from build123d import *

# Parameters (mm, degrees)
CUT_EXTRUDE1_DEPTH = 0.75
FILLET1_R          = 0.125
WRAP1_START        = -0.125
WRAP1_DEPTH        = 0.125


# Read off the part's stored shape, not the designer's step: Wrap1
with BuildPart() as part:
    # Sketch1 → Revolve1 (revolve)
    with BuildSketch(Plane(origin=(0, 0, 0), x_dir=(0, 0, -1), z_dir=(1, 0, 0)), mode=Mode.PRIVATE) as revolve1_sk:
        with BuildLine():
            Line((0, 1.5), (-1.75, 1.5))
            ThreePointArc((-1.75, 1.5), (-2.334912942, 0.942930354), (-2.75, 0.25))
            Line((-2.75, 0.25), (-2.605662433, 0))
            Line((-2.605662433, 0), (-1.5, 0))
            Line((-1.5, 0), (-1.5, -6))
            Line((-1.5, -6), (0, -6))
            Line((0, -6), (0, 1.5))
        make_face()
    revolve(revolve1_sk.sketch.rotate(Axis((0, -6, 0), (0, 1, 0)), 180), axis=Axis((0, -6, 0), (0, 1, 0)))

    # Sketch2 → Cut-Extrude1 (cut)
    with BuildSketch(Plane(origin=(0, 1.5, 0), x_dir=(1, 0, 0), z_dir=(0, 1, 0))):
        Polygon((0, 1.154700538), (-1, 0.577350269), (-1, -0.577350269), (0, -1.154700538), (1, -0.577350269), (1, 0.577350269), align=None)
    extrude(amount=-CUT_EXTRUDE1_DEPTH, mode=Mode.SUBTRACT)

    # Fillet1
    fillet1_edges = [part.edges().sort_by_distance(p)[0] for p in [
        (0.5, 1.5, -0.866025404),
        (-0.5, 1.5, -0.866025404),
        (-1, 1.5, 0),
        (-0.5, 1.5, 0.866025404),
        (0.5, 1.5, 0.866025404),
        (1, 1.5, 0),
        (0, 1.5, 1.75),
    ]]
    fillet(fillet1_edges, radius=FILLET1_R)

    # Wrap1 outline → Wrap1 (cut)
    with BuildSketch(Plane(origin=(0, 0.75, 0), x_dir=(1, 0, 0), z_dir=(0, 1, 0)).offset(WRAP1_START)):
        with BuildLine():
            add(Edge.make_bspline(
                [(-0.537455829, 0.145072229), (-0.537366548, 0.15735919), (-0.537194747, 0.181002472), (-0.536236546, 0.215136123), (-0.534510696, 0.246473554), (-0.531857696, 0.275057496), (-0.528751002, 0.300937263), (-0.524861231, 0.324098842), (-0.520025531, 0.344486675), (-0.512963856, 0.367808475), (-0.501673714, 0.39403328), (-0.484042302, 0.422215735), (-0.462961845, 0.447719467), (-0.43819726, 0.469796385), (-0.410438674, 0.48826361), (-0.379753396, 0.501330341), (-0.346770262, 0.509472114), (-0.323962243, 0.510388658), (-0.312295573, 0.510857485)],
                knots=[0, 0, 0, 0, 0.075666503, 0.145601872, 0.210267314, 0.268902852, 0.322354979, 0.370758742, 0.413447068, 0.451298193, 0.520734923, 0.588514213, 0.655379256, 0.723813985, 0.792131248, 0.85973193, 0.928250616, 1, 1, 1, 1], degree=3))
            Line((-0.537455829, 0.145072229), (-0.537455829, -0.527604053))
            Line((-0.537455829, -0.527604053), (-0.460532752, -0.527604053))
            Line((-0.460532752, -0.527604053), (-0.460532752, 0.137460049))
            add(Edge.make_bspline(
                [(-0.447712239, 0.305328639), (-0.448774545, 0.301469619), (-0.451134212, 0.292897693), (-0.453525545, 0.278533298), (-0.455753975, 0.261566558), (-0.457491806, 0.241915402), (-0.458861613, 0.219538201), (-0.459832928, 0.194491685), (-0.460431178, 0.166843342), (-0.460497896, 0.147543183), (-0.460532752, 0.137460049)],
                knots=[0, 0, 0, 0, 0.071102967, 0.157938928, 0.258486703, 0.375288845, 0.508476997, 0.656953648, 0.820779591, 1, 1, 1, 1], degree=3))
            add(Edge.make_bspline(
                [(-0.310292367, 0.421113895), (-0.317674297, 0.420714803), (-0.332400851, 0.419918636), (-0.353965955, 0.413875353), (-0.374511474, 0.403804365), (-0.393760239, 0.390026559), (-0.411220155, 0.372905819), (-0.426330799, 0.352966004), (-0.438683838, 0.330213781), (-0.444651659, 0.313764569), (-0.447712239, 0.305328639)],
                knots=[0, 0, 0, 0, 0.115143072, 0.229704239, 0.346728965, 0.47082069, 0.597615275, 0.727089869, 0.860038825, 1, 1, 1, 1], degree=3))
            add(Edge.make_bspline(
                [(-0.17848147, 0.261057806), (-0.178952566, 0.271974178), (-0.179864172, 0.293098195), (-0.186637459, 0.323530756), (-0.198777604, 0.350930356), (-0.212261145, 0.371485038), (-0.225066026, 0.38586534), (-0.235235588, 0.395399384), (-0.246252738, 0.403200746), (-0.257654824, 0.410013084), (-0.269995595, 0.414921405), (-0.282862679, 0.418632696), (-0.296413152, 0.420560449), (-0.305613195, 0.420927309), (-0.310292367, 0.421113895)],
                knots=[0, 0, 0, 0, 0.141583044, 0.273974039, 0.401600231, 0.528456794, 0.591043942, 0.651122908, 0.708825408, 0.765880537, 0.822988251, 0.880580103, 0.939262648, 1, 1, 1, 1], degree=3))
            add(Edge.make_bspline(
                [(-0.340941406, 0.087780562), (-0.334988303, 0.08792105), (-0.323299062, 0.088196907), (-0.306225523, 0.090764835), (-0.289888322, 0.094368098), (-0.274654087, 0.100137271), (-0.260174408, 0.107124777), (-0.24682212, 0.11601785), (-0.234254323, 0.126336142), (-0.222711003, 0.138095802), (-0.212416341, 0.151054166), (-0.203323514, 0.164708223), (-0.195692258, 0.179095557), (-0.189162431, 0.194099224), (-0.184457799, 0.209936522), (-0.181072867, 0.226359939), (-0.178698712, 0.243427453), (-0.178554801, 0.255106579), (-0.17848147, 0.261057806)],
                knots=[0, 0, 0, 0, 0.067065692, 0.131687113, 0.194317921, 0.255289037, 0.314878218, 0.375218702, 0.435653028, 0.497934511, 0.56059698, 0.621980302, 0.682601877, 0.743985199, 0.806139168, 0.868443394, 0.932963888, 1, 1, 1, 1], degree=3))
            Line((-0.340941406, 0.087780562), (-0.357968649, 0.087780562))
            Line((-0.357968649, 0.087780562), (-0.357968649, -0.014783541))
            add(Edge.make_bspline(
                [(-0.152840444, -0.246153733), (-0.152991921, -0.237935238), (-0.153288163, -0.221862292), (-0.155672785, -0.198335348), (-0.159894598, -0.176034257), (-0.165736265, -0.154867378), (-0.173053307, -0.13483662), (-0.182215246, -0.116043494), (-0.192787882, -0.098300128), (-0.20519576, -0.081953022), (-0.21910276, -0.067000398), (-0.234429011, -0.053697294), (-0.25160782, -0.04265632), (-0.269991613, -0.033131715), (-0.29004854, -0.025867397), (-0.311286964, -0.019869429), (-0.334167811, -0.016416131), (-0.349879854, -0.015338382), (-0.357968649, -0.014783541)],
                knots=[0, 0, 0, 0, 0.070899124, 0.138657723, 0.203740428, 0.266496883, 0.327925022, 0.387445969, 0.44662859, 0.505853257, 0.564143059, 0.622569358, 0.680413321, 0.739931479, 0.800819634, 0.864131594, 0.930052902, 1, 1, 1, 1], degree=3))
            add(Edge.make_bspline(
                [(-0.309891726, -0.450680977), (-0.304334961, -0.450571211), (-0.293413044, -0.450355466), (-0.277514036, -0.447340483), (-0.262286727, -0.442989313), (-0.247781817, -0.436676481), (-0.233907442, -0.428733085), (-0.221051475, -0.418678171), (-0.208664071, -0.407189838), (-0.197187775, -0.393882067), (-0.186871623, -0.37903336), (-0.17755536, -0.363253667), (-0.169907305, -0.346235338), (-0.163848892, -0.328206631), (-0.158625475, -0.30926113), (-0.155449196, -0.289102842), (-0.15305503, -0.26797937), (-0.152912733, -0.253506267), (-0.152840444, -0.246153733)],
                knots=[0, 0, 0, 0, 0.057830355, 0.113666545, 0.168061557, 0.222616608, 0.278122197, 0.334218011, 0.392319921, 0.453992458, 0.516935927, 0.58055674, 0.644719566, 0.710965936, 0.778658745, 0.849251577, 0.923417744, 1, 1, 1, 1], degree=3))
            add(Edge.make_bspline(
                [(-0.409250701, -0.417427771), (-0.40035509, -0.422552084), (-0.383473121, -0.432276934), (-0.357561529, -0.44229785), (-0.333383308, -0.449497533), (-0.317482442, -0.450298576), (-0.309891726, -0.450680977)],
                knots=[0, 0, 0, 0, 0.290177362, 0.550694617, 0.785511707, 1, 1, 1, 1], degree=3))
            Line((-0.409250701, -0.417427771), (-0.409250701, -0.507371682))
            add(Edge.make_bspline(
                [(-0.298273137, -0.540424566), (-0.308861639, -0.540097242), (-0.329301798, -0.539465371), (-0.358664913, -0.532954409), (-0.385682425, -0.522833546), (-0.401463988, -0.512480121), (-0.409250701, -0.507371682)],
                knots=[0, 0, 0, 0, 0.269471748, 0.52019112, 0.763259579, 1, 1, 1, 1], degree=3))
            add(Edge.make_bspline(
                [(-0.075917367, -0.249759502), (-0.076128163, -0.26018073), (-0.076541077, -0.280594276), (-0.079227651, -0.310491914), (-0.084396107, -0.33890103), (-0.091033777, -0.365960134), (-0.09992887, -0.391457717), (-0.110563094, -0.41559927), (-0.123397597, -0.438155636), (-0.137962217, -0.459132621), (-0.153934421, -0.478163377), (-0.171095941, -0.494958486), (-0.189740067, -0.508821331), (-0.209271063, -0.520337979), (-0.2298646, -0.529505832), (-0.251686582, -0.535889962), (-0.274626983, -0.539804561), (-0.290311376, -0.540215808), (-0.298273137, -0.540424566)],
                knots=[0, 0, 0, 0, 0.076485505, 0.149823073, 0.219996399, 0.288217649, 0.354082023, 0.417919027, 0.481558234, 0.544225908, 0.605087621, 0.663657146, 0.720011753, 0.77514507, 0.829777395, 0.884976008, 0.941611157, 1, 1, 1, 1], degree=3))
            add(Edge.make_bspline(
                [(-0.194707432, 0.00885428), (-0.185532098, 0.002246917), (-0.167142487, -0.010995852), (-0.14356067, -0.035865532), (-0.123015599, -0.064046821), (-0.106173919, -0.095826321), (-0.092429948, -0.130510752), (-0.082995533, -0.168026939), (-0.077008082, -0.208034101), (-0.076287996, -0.23558107), (-0.075917367, -0.249759502)],
                knots=[0, 0, 0, 0, 0.114174048, 0.228832702, 0.344903554, 0.466103946, 0.591676048, 0.72144281, 0.856626542, 1, 1, 1, 1], degree=3))
            add(Edge.make_bspline(
                [(-0.273032752, 0.036899152), (-0.264977593, 0.035253476), (-0.249714467, 0.032135208), (-0.228666305, 0.025295577), (-0.210172583, 0.018341569), (-0.199638474, 0.011879289), (-0.194707432, 0.00885428)],
                knots=[0, 0, 0, 0, 0.294434237, 0.557901696, 0.79305271, 1, 1, 1, 1], degree=3))
            add(Edge.make_bspline(
                [(-0.200917367, 0.061939216), (-0.205600715, 0.059219735), (-0.215469689, 0.053489114), (-0.232413767, 0.046806913), (-0.251771921, 0.040993346), (-0.265723651, 0.038306664), (-0.273032752, 0.036899152)],
                knots=[0, 0, 0, 0, 0.211315364, 0.445293882, 0.709397831, 1, 1, 1, 1], degree=3))
            add(Edge.make_bspline(
                [(-0.101558393, 0.265064216), (-0.101829728, 0.254158186), (-0.102360461, 0.23282596), (-0.107582885, 0.201794643), (-0.115635878, 0.172523389), (-0.127393107, 0.145424978), (-0.141807851, 0.120566799), (-0.158666737, 0.09801557), (-0.178511599, 0.078390972), (-0.193428545, 0.067437991), (-0.200917367, 0.061939216)],
                knots=[0, 0, 0, 0, 0.138734507, 0.271365083, 0.399463796, 0.524371928, 0.64626696, 0.764603187, 0.881822663, 1, 1, 1, 1], degree=3))
            add(Edge.make_bspline(
                [(-0.312295573, 0.510857485), (-0.304601721, 0.510709635), (-0.289468193, 0.510418818), (-0.267407867, 0.506806308), (-0.246411552, 0.501505665), (-0.226632783, 0.49383833), (-0.208041676, 0.483900131), (-0.190537128, 0.47184286), (-0.174217748, 0.457507541), (-0.159329374, 0.44106616), (-0.145724285, 0.423136003), (-0.133914037, 0.403846519), (-0.123827558, 0.383480477), (-0.115525112, 0.361982783), (-0.109489008, 0.339238969), (-0.104721569, 0.315513437), (-0.102229905, 0.290624502), (-0.101784813, 0.273682609), (-0.101558393, 0.265064216)],
                knots=[0, 0, 0, 0, 0.063537388, 0.124975739, 0.184284437, 0.242302503, 0.299838056, 0.35817297, 0.417627897, 0.478966986, 0.541230446, 0.60342781, 0.66563497, 0.728883988, 0.793562004, 0.859921094, 0.928741429, 1, 1, 1, 1], degree=3))
        make_face()
        Polygon((0.565629107, -0.527604053), (0.583056992, -0.527604053), (0.583056992, 0.472395947), (0.506133915, 0.472395947), (0.506133915, -0.290224246), (-0.016101662, 0.472395947), (-0.032327624, 0.472395947), (-0.032327624, -0.527604053), (0.044595453, -0.527604053), (0.044595453, 0.233012934), align=None)
        Polygon((0.095877504, 0.741626716), (0.244315004, 0.574960049), (0.318633915, 0.574960049), (0.467672376, 0.741626716), (0.350885517, 0.741626716), (0.280172376, 0.662700434), (0.212664363, 0.741626716), align=None)
    extrude(amount=WRAP1_DEPTH, mode=Mode.SUBTRACT)


solid = part.part
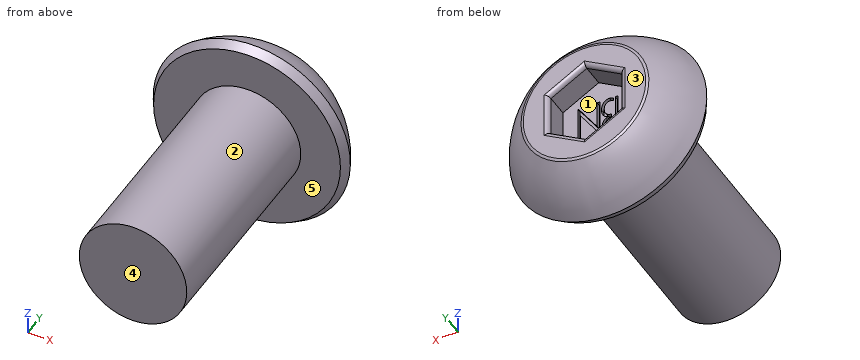
Design review of the part built by this model. Coordinates are the model's own, in mm. Face numbers are marked on the shaded views. A direction names the side the tool comes from. Round coordinates to 2 decimals unless told otherwise and drop trailing zeros. Write each loop counter-clockwise with the first axis right and the second up, starting at its lowest first coordinate (ties: lowest second). Pieces come first, ordered by that corner, then holes. Notation, with made-up numbers: (62, -9) - (66, -9) arc R22 cw to (66, 7) - close; hole circle Ø11 at (-21.5, 22.5). An arc over 180 degrees is marked (long way). Use a Markdown table: item, result. Add a question column.
1. Clearance check with flat-ended pins moving along their axes: pin 1 (2 mm diameter, centred on y = 0.5, z = 0.5, fed in from +X); pin 2 (0.5 mm diameter, centred on x = 0.5, z = 0, fed in from +Y); pin 3 (3 mm diameter, centred on y = -2, z = 1.5, fed in from -X); pin 4 (0.7 mm diameter, centred on y = 1, z = -0.5, fed in from +X). State where each tip first meets the part, or that it passes through.
2. Wall thickness on probe 1 along Y at (x, z) = (0, 0) (3 decimals); probe 2 along X at (y, z) = (1, -0.1); probe 3 along Y at (x, z) = (0.85, 0.55): over which ranges is each line inside the solid? List them lowest first.
3. Mouldability with a two-part tool opening along Z and no side actions: class the marked faces 1, 2 and 3 as +Z half, -Z half, draft (parallel to the pull), parting line (faces both ways), or undercut.
4. We need section A-A (y = -3). State the section outline as (x, z) points, then the cut area to 3 significant figures.
5. For the marked faces 4 and 5, list the 3-axis set-ups (+Z, -Z, +X, -X, +Y, -Y) from which the entire face can be reached by the end or side of a thin tool; tool diameter is ignored.
Output:
| question | item | result |
|---|---|---|
| 1 | pin 1 | stops at x = 2.75 |
| 1 | pin 2 | stops at y = 0.75 |
| 1 | pin 3 | stops at x = -1.5 |
| 1 | pin 4 | stops at x = 2.5 |
| 2 | probe 1 | y = -6 to 0.625 |
| 2 | probe 2 | x = -2.29 to -1, 1 to 2.29 |
| 2 | probe 3 | y = -6 to 0.75 |
| 3 | face 1 | undercut |
| 3 | face 2 | parting line |
| 3 | face 3 | draft |
| 4 | outline | circle Ø3 at (0, 0) |
| 4 | area | 7.07 mm2 |
| 5 | face 4 | +Z, -Z, +X, -X, -Y |
| 5 | face 5 | -Y |
